Read the model definition and answer for the solid it produces. Units are mm, in the model's axes. A direction names the side the tool comes from. Round coordinates to 2 decimals unless told otherwise and drop trailing zeros. Order: outer loops, then holes, each group sorted by start corner. A loop starts at its lowest first (then second) coordinate and runs counter-clockwise, first axis right, second up. Notation, with made-up numbers: (12, 67.5) - (47, 67.5) arc R28 ccw to (47, 87.5) - close; hole circle Ø11 at (4, 70). An arc over 180 degrees is marked (long way). Answer as a JSON object with one key per item and string values. Group by question number.
Q1. The mould has two halves that part along Y. Classify faces 1 (the flat face through (0, 18, 1)), 2 (the flat face through (20, 0, 0)), 3 (the cylindrical face through (-16.18, 16.08, 0.79)): pulls with the +Y half, pulls with the -Y half, needs draft (parallel to the pull), parting line crosses it, or undercut.
Q2. Consider line 1 (Y direction, x = 15, z = 0.95); line 2 (Y direction, x = 0, z = 14.25); line 3 (Z direction, x = 2.5, y = 0.5). Determine where each line is inside the solid, lowest interval first.
Q3. A cutting plane is placed at C-C on z = 3. Determine the outline of the cut face in (x, y), and give its area (3 significant figures).
Q4. A cutting plane is placed at D-D on z = 11.5. Determine the outline of the cut face in (x, y), and give its area (3 significant figures).
Q5. Given pin 1 Ø2.5 at (y, z) = (16, -1.5) entering from +X; pin 2 Ø2 at (x, z) = (-16, -1.5) entering from +Y; pin 3 Ø1 at (x, z) = (-2.5, 7.5) entering from +Y; pin 4 Ø1.9 at (x, y) = (-15, -15) entering from -Z, each flat-ended and moving along its own axis, determine where each tip first touches the part or whether it passes through.
Q6. A cutting plane is placed at A-A on z = -0.5. Determine the outline of the cut face in (x, y), and give its area (3 significant figures).
Q7. A tool of negligible diameter and unlimited length cuts with its end or side. For faces 4 (the cylindrical face through (-14.985, 0.66, 4.121)), 5 (the flat face through (16, -4.35, -2)), 6 (the flat face through (-6.85, 16, -2)), 7 (the flat face through (16, 4.35, -2)), from which of +Z, -Z, +X, -X, +Y, -Y can it reach the whole face along a straight path? Write none if from no direction.
```python
from build123d import *

# Parameters (mm, degrees)
F0_R     = 1.6
F0_W     = 2
F0_H     = 2
F0_W_2   = 13.7
F0_H_2   = 2.9
F0_W_3   = 7.4758231461
F0_H_3   = 8.7
F1_DEPTH = 1.6
F2_DEPTH = 4
F0_W_4   = 3.3
F3_DEPTH = 3.1
F4_DEPTH = 2
F5_R     = 15
F5_R_2   = 10
F6_DEPTH = 8
F7_DEPTH = 12.5
F8_SIZE2 = 2.886741
F8_SIZE  = 4.99999
F5_R_3   = 7
F9_DEPTH = 14.3


# Not quite as in the source:
# - a fillet or chamfer is up to 0.001 mm smaller than in the source, because OpenCascade refuses the exact size


with BuildPart() as f1:
    # F0 (on Top) → F1 (new body)
    with BuildSketch(Plane.XY):
        with BuildLine():
            Line((-18, -18), (18, -18))
            Line((18, -18), (18, -4.35))
            Line((18, -4.35), (10.5241768539, -4.35))
            Line((10.5241768539, -4.35), (10.5241768539, 4.35))
            Line((10.5241768539, 4.35), (18, 4.35))
            Line((18, 4.35), (18, 9.5))
            ThreePointArc((18, 9.5), (17, 10.5), (18, 11.5))
            Line((18, 11.5), (18, 18))
            Line((18, 18), (-18, 18))
            Line((-18, 18), (-18, -18))
        make_face()
        with Locations((-15, -15)):
            Circle(F0_R, mode=Mode.SUBTRACT)
        with Locations((-15.5, -10.5)):
            Rectangle(F0_W, F0_H, mode=Mode.SUBTRACT)
        with Locations((15, -15)):
            Circle(F0_R, mode=Mode.SUBTRACT)
        with Locations((-15, 15)):
            Circle(F0_R, mode=Mode.SUBTRACT)
        with Locations((0, 15.9)):
            Rectangle(F0_W_2, F0_H_2, mode=Mode.SUBTRACT)
        with Locations((15, 15)):
            Circle(F0_R, mode=Mode.SUBTRACT)
        with Locations((0, 15.9)):
            Rectangle(F0_W_2, F0_H_2)
        with Locations((-15.5, -10.5)):
            Rectangle(F0_W, F0_H)
        with Locations((14.2620884269, 0)):
            Rectangle(F0_W_3, F0_H_3)
    extrude(amount=F1_DEPTH)

    # F0 (on Top) → F2 (join)
    with BuildSketch(Plane.XY):
        with Locations((0, 15.9)):
            Rectangle(F0_W_2, F0_H_2)
    extrude(amount=-F2_DEPTH)

    # F0 (on Top) → F3 (join)
    with BuildSketch(Plane.XY):
        with Locations((19.65, 0)):
            Rectangle(F0_W_4, F0_H_3)
        with Locations((14.2620884269, 0)):
            Rectangle(F0_W_3, F0_H_3)
    extrude(amount=-F3_DEPTH)

    # F0 (on Top) → F4 (join)
    with BuildSketch(Plane.XY):
        with Locations((-15.5, -10.5)):
            Rectangle(F0_W, F0_H)
    extrude(amount=-F4_DEPTH)

    # F5 (on face) → F6 (join)
    with BuildSketch(Plane.XY.offset(1.6)):
        Circle(F5_R)
        Circle(F5_R_2, mode=Mode.SUBTRACT)
    extrude(amount=F6_DEPTH)

    # F7 (add): a face of the model
    f7_faces = [f1.faces().sort_by_distance(p)[0] for p in [
        (0, 0, 1.6),
    ]]
    extrude(f7_faces, amount=F7_DEPTH)

    # F8 (size 5 and 2.8867513459 in the source; OpenCascade refuses exactly that, so slightly less here)
    f8_edges = [f1.edges().sort_by_distance(p)[0] for p in [
        (-15, 0, 9.6),
    ]]
    f8_side = f1.faces().sort_by_distance((-14.575736, 0, 9.6))[0]
    chamfer(f8_edges, length=F8_SIZE, length2=F8_SIZE2, reference=f8_side)

    # F5 (on face) → F9 (join)
    with BuildSketch(Plane.XY.offset(1.6)):
        Circle(F5_R_3)
    extrude(amount=F9_DEPTH)


solid = f1.part
```
Result set:
{
 "1": {"face 1": "pulls with the +Y half", "face 2": "needs draft", "face 3": "undercut"},
 "2": {"line 1": "y = -18 to -16.6, -13.4 to 13.4, 16.6 to 18", "line 2": "y = -7 to 7", "line 3": "z = 0 to 15.9"},
 "3": {"outline": "circle Ø30 at (0, 0)", "area": "707 mm²"},
 "4": {"outline": "circle Ø20 at (0, 0)", "area": "314 mm²"},
 "5": {"pin 1": "stops at x = 6.85", "pin 2": "stops at y = -9.5", "pin 3": "stops at y = 14.29", "pin 4": "passes through"},
 "6": {"outline": "(-16.5, -11.5) - (-14.5, -11.5) - (-14.5, -9.5) - (-16.5, -9.5) - close; (-6.85, 14.45) - (6.85, 14.45) - (6.85, 17.35) - (-6.85, 17.35) - close; (10.52, -4.35) - (21.3, -4.35) - (21.3, 4.35) - (10.52, 4.35) - close", "area": "137 mm²"},
 "7": {"face 4": "+Z", "face 5": "-Z, +X, -X, -Y", "face 6": "-Z, -X, +Y, -Y", "face 7": "-Z, +X, -X, +Y"}
}
